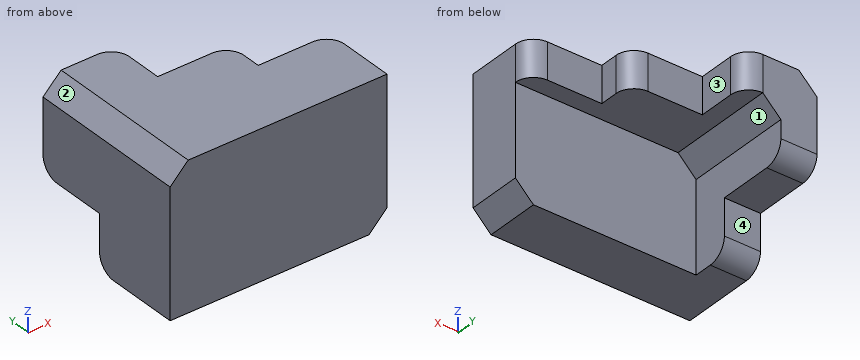
```python
from build123d import *

# Parameters (mm, degrees)
SKETCH1_W           = 60
SKETCH1_H           = 40
BOSS_EXTRUDE1_DEPTH = 45
CUT_EXTRUDE1_START  = 45
SKETCH1_3_W         = 50
SKETCH1_3_H         = 30
CUT_EXTRUDE1_DEPTH  = 30
SKETCH2_W           = 40
SKETCH2_H           = 15
SKETCH2_W_2         = 20
SKETCH2_H_2         = 10
CUT_EXTRUDE2_DEPTH  = 30
SKETCH3_W           = 15
SKETCH3_H           = 20
CUT_EXTRUDE3_DEPTH  = 30
FILLET1_R           = 5
CHAMFER2_SIZE       = 5


with BuildPart() as part:
    # Sketch1 → Boss-Extrude1 (new body)
    with BuildSketch(Plane(origin=(0, 0, 0), x_dir=(1, 0, 0), z_dir=(0, 1, 0))):
        with Locations((30, 20)):
            Rectangle(SKETCH1_W, SKETCH1_H)
    extrude(amount=BOSS_EXTRUDE1_DEPTH)

    # Sketch1<3> → Cut-Extrude1 (cut)
    with BuildSketch(Plane(origin=(0, 0, 0), x_dir=(1, 0, 0), z_dir=(0, 1, 0)).offset(CUT_EXTRUDE1_START)):
        with Locations((35, 25)):
            Rectangle(SKETCH1_3_W, SKETCH1_3_H)
    extrude(amount=-CUT_EXTRUDE1_DEPTH, mode=Mode.SUBTRACT)

    # Sketch2 → Cut-Extrude2 (cut)
    with BuildSketch(Plane.XY):
        with Locations((40, 37.5)):
            Rectangle(SKETCH2_W, SKETCH2_H)
        with Locations((50, 25)):
            Rectangle(SKETCH2_W_2, SKETCH2_H_2)
    extrude(amount=-CUT_EXTRUDE2_DEPTH, mode=Mode.SUBTRACT)

    # Sketch3 → Cut-Extrude3 (cut)
    with BuildSketch(Plane(origin=(0, 0, 0), x_dir=(0, 0, -1), z_dir=(1, 0, 0))):
        with Locations((32.5, 35)):
            Rectangle(SKETCH3_W, SKETCH3_H)
    extrude(amount=CUT_EXTRUDE3_DEPTH, mode=Mode.SUBTRACT)

    # Fillet1
    fillet1_edges = [part.edges().sort_by_distance(p)[0] for p in [
        (5, 25, -40),
        (5, 45, -25),
        (20, 45, -5),
        (40, 30, -5),
        (60, 20, -5),
    ]]
    fillet(fillet1_edges, radius=FILLET1_R)

    # Chamfer2
    chamfer2_edges = [part.edges().sort_by_distance(p)[0] for p in [
        (10, 30, -10),
        (60, 7.5, -40),
        (0, 22.5, 0),
    ]]
    chamfer(chamfer2_edges, length=CHAMFER2_SIZE)


solid = part.part
```
Source: CAD feature listing. Evaluate the final solid. Frame: model axes, mm. Face numbers are marked on the shaded views. A direction names the side the tool comes from. Round coordinates to 2 decimals unless told otherwise and drop trailing zeros. Loops run counter-clockwise (first coordinate to the right, second up) from the corner with the lowest first, then second, coordinate; pieces in that order, holes last. Notation, with made-up numbers: M 22.5,-6.5 L 57.5,-6.5 A25 ccw 57.5,9.5 Z; hole C 22.25,57.25 d3. An arc over 180 degrees is marked long. Use a Markdown table: item, result. Add a question column.
1. Cut plane A-A, the plane y = 39. Output: boundary loops of the cut face in (x, z), and give its area (3 significant figures).
2. Cut plane C-C, the plane x = 18. Output: boundary loops of the cut face in (y, z), and give its area (3 significant figures).
3. Ray query, line 1 along Y through (x, z) = (27, -18); line 2 along X through (y, z) = (38.5, -9.5); line 3 along X through (y, z) = (32, -22). Return the intervals inside material, ascending. Write a range as [from, to].
4. Cut plane D-D, the plane y = 28.5. Output: boundary loops of the cut face in (x, z), and give its area (3 significant figures).
5. Cut plane B-B, the plane z = -17.5. Output: boundary loops of the cut face in (x, y), and give its area (3 significant figures).
6. Contact query for flat-ended pins moving along their axis: pin 1 (12.5 mm diameter, centred on y = 24.5, z = -25, fed in from +X); pin 2 (3 mm diameter, centred on x = 44.5, z = -6.5, fed in from +Y); pin 3 (5 mm diameter, centred on x = 31, z = -6, fed in from +Y). Output: stop coordinate, or through.
7. Set-up query: the marked faces 1, 2, 3 and 4. Return all of +Z, -Z, +X, -X, +Y, -Y with unobstructed straight access to the full face (end or side cutting, diameter ignored); none if empty.
Solution:
| question | item | result |
|---|---|---|
| 1 | outline | M 0,-25 L 10,-25 L 10,-15 L 15,-10 L 20,-10 L 20,0 L 5,0 L 0,-5 Z |
| 1 | area | 350 mm2 |
| 2 | outline | M 0,-40 L 15,-40 L 15,-10 L 44,-10 L 44,0 L 0,0 Z |
| 2 | area | 890 mm2 |
| 3 | line 1 | y = [0, 15] |
| 3 | line 2 | x = [0, 20] |
| 3 | line 3 | x = [0, 10] |
| 4 | outline | M 0,-25 L 10,-25 L 10,-15 L 15,-10 L 38.57,-10 L 38.57,0 L 5,0 L 0,-5 Z |
| 4 | area | 536 mm2 |
| 5 | outline | M 0,0 L 60,0 L 60,15 L 10,15 L 10,45 L 0,45 Z |
| 5 | area | 1,200 mm2 |
| 6 | pin 1 | stops at x = 10 |
| 6 | pin 2 | stops at y = 20 |
| 6 | pin 3 | stops at y = 30 |
| 7 | face 1 | -Z, +X, +Y |
| 7 | face 2 | +Z, -X, +Y, -Y |
| 7 | face 3 | +Z, -Z, +X, +Y |
| 7 | face 4 | -Z, +X, -X, +Y |
